```python
from build123d import *

# Parameters (mm, degrees)
SKETCH7_W               = 4.7625
SKETCH7_H               = 2.12122512
BOSS_EXTRUDE2_DEPTH     = 130.175
BOSS_EXTRUDE3_DEPTH     = 130.175
BOSS_EXTRUDE4_DEPTH     = 130.175
CUT_EXTRUDE1_DEPTH      = 66.021233396
CUT_EXTRUDE1_DEPTH_BACK = 36.912098974


with BuildPart() as part:
    # Sketch7 → Boss-Extrude2 (new body, symmetric)
    with BuildSketch(Plane.XY):
        with Locations((-4.92125, -2.560612608)):
            Rectangle(SKETCH7_W, SKETCH7_H)
    extrude(amount=BOSS_EXTRUDE2_DEPTH, both=True)



with BuildPart() as body_2:
    # Sketch8 → Boss-Extrude3 (new body, symmetric)
    with BuildSketch(Plane.XY):
        Polygon((2.569038147, 1.449704502), (4.950288147, 5.574150487), (6.787322988, 4.513537927), (4.406072988, 0.389091942), align=None)
    extrude(amount=BOSS_EXTRUDE3_DEPTH, both=True)


with BuildPart() as part_1:
    add(part.part)

    add(body_2.part)  # Boss-Extrude4 merges body 2
    # Sketch11 → Boss-Extrude4 (add, symmetric)
    with BuildSketch(Plane.XY):
        with BuildLine():
            Line((-2.54, -1.500000048), (-7.3025, -1.500000048))
            Line((-7.3025, -1.500000048), (-7.3025, -3.621225168))
            Line((-7.3025, -3.621225168), (-2.54, -3.621225168))
            ThreePointArc((-2.54, -3.621225168), (1.47031711, -2.546663937), (4.406072988, 0.389091942))
            Line((4.406072988, 0.389091942), (6.787322988, 4.513537927))
            Line((6.787322988, 4.513537927), (4.950288147, 5.574150487))
            Line((4.950288147, 5.574150487), (2.569038147, 1.449704502))
            Line((2.569038147, 1.449704502), (-0.029038147, 2.94970455))
            ThreePointArc((-0.029038147, 2.94970455), (-1.090295498, 1.888447198), (-2.54, 1.500000048))
            Line((-2.54, 1.500000048), (-2.54, -1.500000048))
        make_face()
    extrude(amount=BOSS_EXTRUDE4_DEPTH, both=True)

    # Sketch17 → Cut-Extrude1 (cut, two sides)
    with BuildSketch(Plane(origin=(0, 0, 46.419822061), x_dir=(-0.666666667, -0.577350269, 0.471404521), z_dir=(0.471404521, -0.816496581, -0.333333333))) as cut_extrude1_sk:
        Polygon((304.8, 0), (0, 0), (-152.4, -263.964543073), (-304.8, 0), (-152.4, 263.964543073), (152.4, 263.964543073), align=None)
    extrude(amount=CUT_EXTRUDE1_DEPTH, mode=Mode.SUBTRACT)
    extrude(cut_extrude1_sk.sketch, amount=-CUT_EXTRUDE1_DEPTH_BACK, mode=Mode.SUBTRACT)


solid = part_1.part
```
Could you check a few things on this model? Use its own coordinates, in mm. A direction names the side the tool comes from. Round coordinates to 2 decimals unless told otherwise and drop trailing zeros. Loops run counter-clockwise (first coordinate to the right, second up) from the corner with the lowest first, then second, coordinate; pieces in that order, holes last. Notation, with made-up numbers: (68, -38.5) -> (117, -38.5) arc R20 cw to (117, -20.5) -> close; hole circle Ø7 at (10, 34.5). An arc over 180 degrees is marked (long way). One line per question, with ' | ' between items.
(1) If we section it at B-B on x = 3.5: List the corners of the cut face in (y, z) for me (3 decimals).
Model answer:
outline: (-0.878, 47.12) -> (3.062, 49.532) -> (3.062, 130.175) -> (-0.878, 130.175) -> close
(2) If we section it at A-A on z = 102.5: List the corners of the cut face in (x, y) for me.
Model answer:
outline: (-7.3, -3.62) -> (-2.54, -3.62) arc R8.02 ccw to (4.41, 0.39) -> (6.79, 4.51) -> (4.95, 5.57) -> (2.57, 1.45) -> (-0.03, 2.95) arc R2.9 cw to (-2.54, 1.5) -> (-2.54, -1.5) -> (-7.3, -1.5) -> close
(3) If I drill on probe 1 along Y at (x, z) = (-5.5, 79.5); probe 2 along Y at (x, z) = (-2.25, 76.5); probe 3 along X at (y, z) = (2.25, 69), over which ranges is the centre line in solid material (lowest first)?
Model answer:
probe 1: y = -3.62 to -1.5 | probe 2: y = -3.62 to 1.51 | probe 3: x = -0.59 to 1.18, 3.03 to 5.48
(4) If we section it at C-C on x = -3.75: List the corners of the cut face in (y, z) for me (3 decimals), and give its area (3 significant figures).
Model answer:
outline: (-3.621, 49.071) -> (-1.5, 49.071) -> (-1.5, 130.175) -> (-3.621, 130.175) -> close | area: 172 mm^2
(5) For faces 5 (the face through (-5, -1.5, 90)), 6 (the face through (-2.649, -1.853, 48.293)), which set-ups out of +Z, -Z, +X, -X, +Y, -Y let a thin tool reach every point of the face, with its end or its side?
Model answer:
face 5: +Z, -Z, -X, +Y | face 6: -Z, -X, +Y, -Y
(6) For pin 1 Ø4 at (x, y) = (3.5, 2.5) entering from -Z; pin 2 Ø1 at (y, z) = (3.5, 63.5) entering from +X; pin 3 Ø5 at (x, z) = (-5.5, 94) entering from +Y, each with a flat end and sliding along its axis, tell me the tip position at first contact or that it passes through.
Model answer:
pin 1: stops at z = 47.77 | pin 2: stops at x = 6.49 | pin 3: stops at y = -1.5
(7) Thinking about a two-plate mould opening in X: for faces 1 (the face through (-1.07, 1.9, 89.26)), 2 (the face through (3.74, 3.48, 89.77)), 3 (the face through (1.29, 2.19, 89.77)), 4 (the face through (0, 0, 130.175)), which applies, released by +X, released by -X, zero draft, split by the parting line, or undercut?
Model answer:
face 1: released by -X | face 2: undercut | face 3: undercut | face 4: zero draft
